```python
from build123d import *

# Parameters (mm, degrees)
SKETCH1_R               = 10
SKETCH1_R_2             = 4
BOSS_EXTRUDE1_DEPTH     = 8
SKETCH2_W               = 0.5
SKETCH2_H               = 17
CUT_EXTRUDE1_DEPTH      = 8
SKETCH3_R               = 2
CUT_EXTRUDE2_DEPTH      = 11
CUT_EXTRUDE2_DEPTH_BACK = 11


with BuildPart() as part:
    # Sketch1 → Boss-Extrude1 (new body)
    with BuildSketch(Plane.XY):
        Circle(SKETCH1_R)
        Circle(SKETCH1_R_2, mode=Mode.SUBTRACT)
    extrude(amount=BOSS_EXTRUDE1_DEPTH)

    # Sketch2 → Cut-Extrude1 (cut)
    with BuildSketch(Plane.XY.offset(8)):
        with Locations((0, 2)):
            Rectangle(SKETCH2_W, SKETCH2_H)
    extrude(amount=-CUT_EXTRUDE1_DEPTH, mode=Mode.SUBTRACT)

    # Sketch3 → Cut-Extrude2 (cut, two sides)
    with BuildSketch(Plane(origin=(0, 0, 0), x_dir=(0, 0, -1), z_dir=(1, 0, 0))) as cut_extrude2_sk:
        with Locations((-4, 7)):
            Circle(SKETCH3_R)
    extrude(amount=CUT_EXTRUDE2_DEPTH, mode=Mode.SUBTRACT)
    extrude(cut_extrude2_sk.sketch, amount=-CUT_EXTRUDE2_DEPTH_BACK, mode=Mode.SUBTRACT)


solid = part.part
```
Could you check a few things on this model? Use its own coordinates, in mm. A direction names the side the tool comes from. Give positions to 0.01 mm unless a question says otherwise; leave off trailing zeros. Order: outer loops, then holes, each group sorted by start corner. A loop starts at its lowest first (then second) coordinate and runs counter-clockwise, first axis right, second up.
Q1. For faces 5 (the cylindrical face through (3, 5, 4)), 6 (the flat face through (0.25, -5, 4)), 7 (the cylindrical face through (-4, 0, 4)), which set-ups out of +Z, -Z, +X, -X, +Y, -Y let a thin tool reach every point of the face, with its end or its side?
Q2. I'm going to push flat-ended pins straight in: P1, Ø1.5, axis at x = -5, z = 1, coming from the -Y side; P2, Ø4, axis at x = 4.5, z = 7, coming from the -Y side; P3, Ø2, axis at y = -5.5, z = 5.5, coming from the +X side; P4, Ø3, axis at y = 7, z = 4, coming from the +X side. Where does each tip first touch, or does it pass through?
Q3. Suppose I cut it at B-B, the plane x = -1.5. Write out the boundary of the cut face in (y, z), and give its area (3 significant figures).
Q4. Suppose I cut it at A-A, the plane y = -6. Write out the boundary of the cut face in (x, z), and give its area (3 significant figures).
Q5. If I drill on line 1 along X through (y, z) = (0, 7.5); line 2 along Y through (x, z) = (3, 2.75); line 3 along Z through (x, y) = (-4.5, 7), over which ranges is the centre line in solid material (lowest first)?
Q6. Suppose I cut it at D-D, the plane z = 4. Write out the boundary of the cut face in (x, y), and give its area (3 significant figures).
Q7. We'd pull the mould along Z, two halves only. Please class faces 1 (the flat face through (4.3, 0.1, 8)), 2 (the cylindrical face through (-3, 5, 4)), 3 (the flat face through (4.3, 0.1, 0)), 4 (the flat face through (-0.25, 5, 3)): +Z half, -Z half, draft (parallel to the pull), parting line (faces both ways), or undercut.
Q8. Suppose I cut it at C-C, the plane z = 6.75. Write out the boundary of the cut face in (x, y), and give its area (3 significant figures).
Solution:
1. face 5: +X, -X
1. face 6: +Z, -Z, +Y
1. face 7: +Z, -Z
2. P1: stops at y = -9.05
2. P2: stops at y = -9.68
2. P3: stops at x = 8.93
2. P4: passes through
3. outline: (-9.89, 0) - (-3.71, 0) - (-3.71, 8) - (-9.89, 8) - close; (3.71, 0) - (9.89, 0) - (9.89, 8) - (3.71, 8) - close; hole circle Ø4 at (7, 4)
3. area: 86.3 mm2
4. outline: (-8, 0) - (-0.25, 0) - (-0.25, 8) - (-8, 8) - close; (0.25, 0) - (8, 0) - (8, 8) - (0.25, 8) - close
4. area: 124 mm2
5. line 1: x = -10 to -4, 4 to 10
5. line 2: y = -9.54 to -2.65, 2.65 to 5.44, 8.56 to 9.54
5. line 3: z = 0 to 2, 6 to 8
6. outline: (-8.66, 5) arc R10 ccw (long way) to (8.66, 5) - (0.25, 5) - (0.25, 3.99) arc R4 cw to (0.25, -3.99) - (0.25, -6.5) - (-0.25, -6.5) - (-0.25, -3.99) arc R4 cw to (-0.25, 3.99) - (-0.25, 5) - close; (-4.36, 9) - (-0.25, 9) - (-0.25, 10) arc R10 ccw to start; (0.25, 9) - (4.36, 9) arc R10 ccw to (0.25, 10) - close
6. area: 206 mm2
7. face 1: +Z half
7. face 2: undercut
7. face 3: -Z half
7. face 4: draft
8. outline: (-0.25, -6.5) - (-0.25, -3.99) arc R4 cw to (-0.25, 3.99) - (-0.25, 10) arc R10 ccw (long way) to (0.25, 10) - (0.25, 3.99) arc R4 cw to (0.25, -3.99) - (0.25, -6.5) - close
8. area: 260 mm2
